from build123d import *

# Parameters (mm, degrees)
F0_W     = 0.5
F0_H     = 9.5
F1_DEPTH = 0.3


with BuildPart() as f1:
    # F0 (on Top) → F1 (new body)
    with BuildSketch(Plane.XY):
        Polygon((5, 5), (-5, 5), (-5, -5), (5, -5), (5, -4.5), align=None)
        Polygon((14.5, -4.5), (5, -4.5), (5, -5), (15, -5), (15, -4.5), align=None)
        with Locations((14.75, 0.25)):
            Rectangle(F0_W, F0_H)
    extrude(amount=F1_DEPTH)


solid = f1.part
Could you check a few things on this model? Use its own coordinates, in mm. Give positions to 0.01 mm unless a question says otherwise; leave off trailing zeros. Order: outer loops, then holes, each group sorted by start corner. A loop starts at its lowest first (then second) coordinate and runs counter-clockwise, first axis right, second up. Notation, with made-up numbers: (24, -10) - (76, -10) arc R24 cw to (76, 21) - close; hole circle Ø6 at (61, -10). An arc over 180 degrees is marked (long way). One line per item, written item: value. Start each with the question number.
1. Imagine slicing it at A-A on y = 1. List the corners of the cut face in (x, z) for me, plus the area to 3 significant figures.
2. Imagine slicing it at B-B on z = 0.1. List the corners of the cut face in (x, y) for me, plus the area to 3 significant figures.
3. Imagine slicing it at C-C on x = 9.5. List the corners of the cut face in (y, z) for me.
4. If I drill on probe 1 along X at (y, z) = (3.75, 0.2); probe 2 along Y at (x, z) = (13, 0.1), over which ranges is the centre line in solid material (lowest first)?
Values:
1. outline: (-5, 0) - (5, 0) - (5, 0.3) - (-5, 0.3) - close; (14.5, 0) - (15, 0) - (15, 0.3) - (14.5, 0.3) - close
1. area: 3.15 mm²
2. outline: (-5, -5) - (15, -5) - (15, 5) - (14.5, 5) - (14.5, -4.5) - (5, -4.5) - (5, 5) - (-5, 5) - close
2. area: 110 mm²
3. outline: (-5, 0) - (-4.5, 0) - (-4.5, 0.3) - (-5, 0.3) - close
4. probe 1: -5 to 5, 14.5 to 15
4. probe 2: -5 to -4.5
